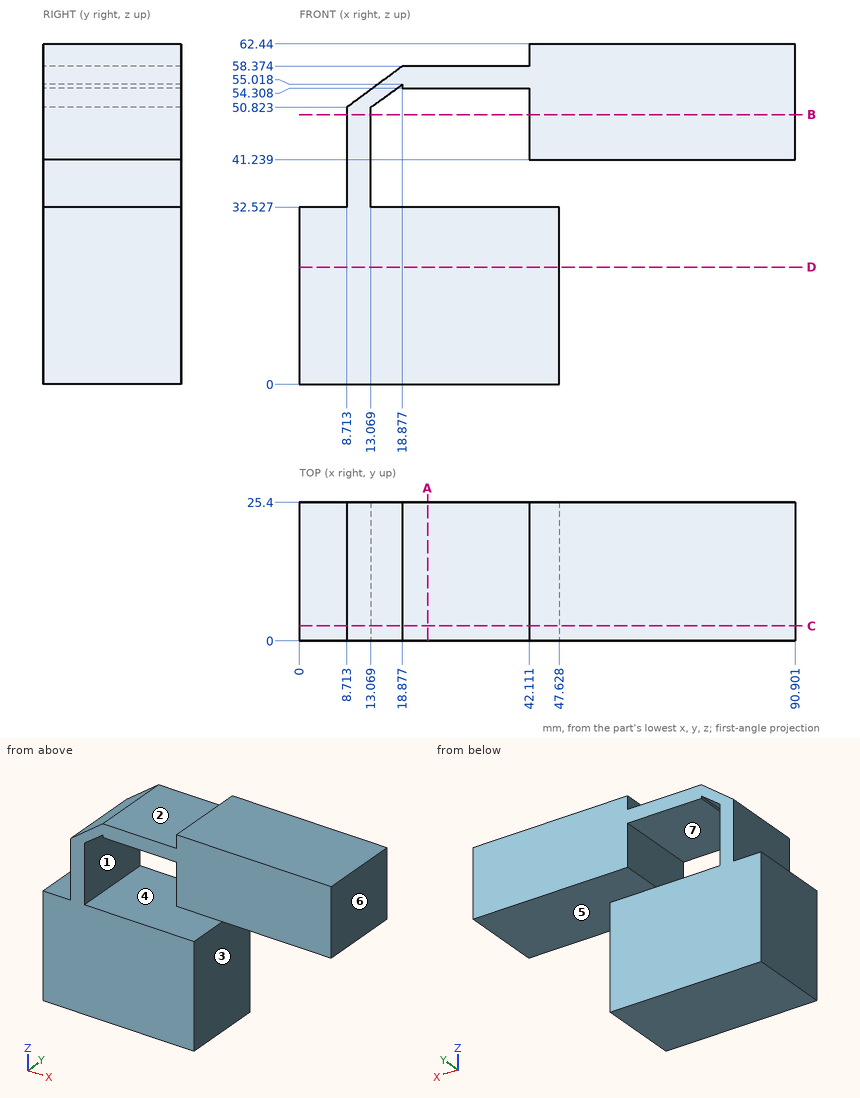
Verification items for this drawing (mm, ordinates from the low corner). A direction names the side the tool comes from. Give positions to 0.01 mm unless a question says otherwise; leave off trailing zeros. Write each loop counter-clockwise with the first axis right and the second up, starting at its lowest first coordinate (ties: lowest second). Pieces come first, ordered by that corner, then holes.
1) Section check A-A, the plane x = 23.5. Record the boundary of the cut face in (y, z).
2) Section check D-D, the plane z = 21.5. Record the boundary of the cut face in (x, y).
3) Material ranges on L1, parallel to Z at x = 34, y = 5.25; L2, parallel to Z at x = 44.5, y = 2; L3, parallel to Z at x = 50, y = 11.5, recorded low to high.
4) Section check B-B, the plane z = 49.5. Record the boundary of the cut face in (x, y).
5) Access from +Z, -Z, +X, -X, +Y, -Y to the whole of each face (thin tool, end or side, straight path). Record for the marked faces 1, 2, 3 and 4.
6) Gauge pin test, flat ends, axial feed: pin 1 (2.5 mm diameter, centred on x = 3.5, y = 15, fed in from +Z); pin 2 (7 mm diameter, centred on x = 35.5, y = 10, fed in from +Z); pin 3 (12.5 mm diameter, centred on x = 67.5, y = 12.5, fed in from -Z). Record the tip position at first contact, or that the pin passes through.
7) Release check for a two-part mould opening along X. For the marked faces 5, 6 and 7 record: pulls with the +X half, pulls with the -X half, needs draft (parallel to the pull), parting line crosses it, or undercut.
8) Section check C-C, the plane y = 2.75. Record the boundary of the cut face in (x, z).
Computed:
1. outline: (0, 0) - (25.4, 0) - (25.4, 32.53) - (0, 32.53) - close; (0, 54.31) - (25.4, 54.31) - (25.4, 58.37) - (0, 58.37) - close
2. outline: (0, 0) - (47.63, 0) - (47.63, 25.4) - (0, 25.4) - close
3. L1: z = 0 to 32.53, 54.31 to 58.37
3. L2: z = 0 to 32.53, 41.24 to 62.44
3. L3: z = 41.24 to 62.44
4. outline: (8.71, 0) - (13.07, 0) - (13.07, 25.4) - (8.71, 25.4) - close; (42.11, 0) - (90.9, 0) - (90.9, 25.4) - (42.11, 25.4) - close
5. face 1: +Y, -Y
5. face 2: +Z, -X, +Y, -Y
5. face 3: -Z, +X, +Y, -Y
5. face 4: +X, +Y, -Y
6. pin 1: stops at z = 32.53
6. pin 2: stops at z = 58.37
6. pin 3: stops at z = 41.24
7. face 5: needs draft
7. face 6: pulls with the +X half
7. face 7: undercut
8. outline: (0, 0) - (47.63, 0) - (47.63, 32.53) - (13.07, 32.53) - (13.07, 50.82) - (18.88, 55.02) - (18.88, 54.31) - (42.11, 54.31) - (42.11, 41.24) - (90.9, 41.24) - (90.9, 62.44) - (42.11, 62.44) - (42.11, 58.37) - (18.88, 58.37) - (8.71, 50.82) - (8.71, 32.53) - (0, 32.53) - close
